Design review of the part shown in the three views and the two pictorial views. Dimensions are in mm from the part's minimum x, y and z. A direction names the side the tool comes from. Coordinates: 2 decimals unless noted, no trailing zeros. Loops run counter-clockwise (first coordinate to the right, second up) from the corner with the lowest first, then second, coordinate; pieces in that order, holes last. Notation, with made-up numbers: (35, -32) - (43, -32) arc R34 cw to (43, 0) - close; hole circle Ø9 at (35.5, -11.75). An arc over 180 degrees is marked (long way). One line per item, written item: value. Start each with the question number.
1. Take a section at A-A, the plane x = 13.5. State the section outline as (y, z) points.
2. For the marked faces 4, 5, 6, 7 and 8, list the 3-axis set-ups (+Z, -Z, +X, -X, +Y, -Y) from which the entire face can be reached by the end or side of a thin tool; tool diameter is ignored.
3. Take a section at C-C, the plane y = 6.5. State the section outline as (x, z) points.
4. Take a section at D-D, the plane x = 6. State the section outline as (y, z) points (1 decimal).
5. Insertion check: pin 1 (6 mm diameter, centred on y = 12, z = 6, fed in from -X); pin 2 (5 mm diameter, centred on y = 3.5, z = 5.5, fed in from +X); pin 3 (1.8 mm diameter, centred on x = 6.5, z = 2.5, fed in from +Y). Each pin has a flat end and moves straight along its axis. Give the tip position at first contact, or say it passes through.
6. The part is to be moulded in two halves that separate along Y. For the marked faces 1, 2 and 3, say which applies: released by +Y, released by -Y, zero draft, split by the parting line, or undercut.
7. To check wall thickness, follow line 1 (Y direction, x = 7.5, z = 10); line 2 (X direction, y = 15, z = 8.25); line 3 (Y direction, x = 26, z = 8). State the ranges of each line that lie inside material, in increasing order. Write a range as from..to.
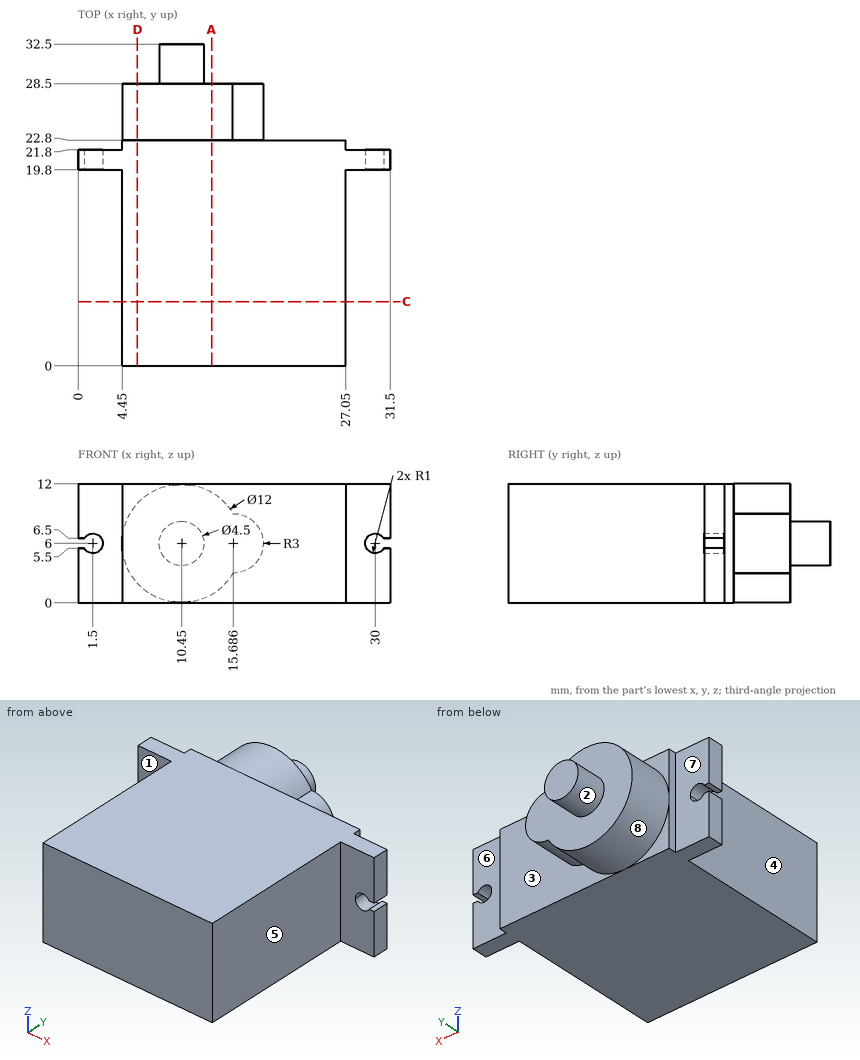
Solutions:
1. outline: (0, 0) - (22.8, 0) - (22.8, 0.83) - (28.5, 0.83) - (28.5, 11.17) - (22.8, 11.17) - (22.8, 12) - (0, 12) - close
2. face 4: +Z, -Z, -X, -Y
2. face 5: +Z, -Z, +X, -Y
2. face 6: +Z, -Z, +X, +Y
2. face 7: +Z, -Z, -X, +Y
2. face 8: +Y
3. outline: (4.45, 0) - (27.05, 0) - (27.05, 12) - (4.45, 12) - close
4. outline: (0, 0) - (22.8, 0) - (22.8, 2) - (28.5, 2) - (28.5, 10) - (22.8, 10) - (22.8, 12) - (0, 12) - close
5. pin 1: x = 4.45
5. pin 2: x = 27.05
5. pin 3: y = 28.5
6. face 1: released by -Y
6. face 2: zero draft
6. face 3: released by +Y
7. line 1: 0..28.5
7. line 2: 4.45..27.05
7. line 3: 0..22.8
